```python
from build123d import *

# Parameters (mm, degrees)
F0_R     = 75.6558411923
F1_DEPTH = 48.514
F2_R     = 5.08


with BuildPart() as f1:
    # F0 (on Top) → F1 (new body)
    with BuildSketch(Plane.XY):
        Circle(F0_R)
        Polygon((0, -69.7530433536), (-46.3102683425, -29.7708865255), (41.9956482947, -29.7708865255), align=None, mode=Mode.SUBTRACT)
        with BuildLine():
            add(Edge.make_bspline(
                [(-21.8607485294, 33.7978675961), (-21.8607485294, 44.4959185344), (-39.0945518587, 45.4823768148)],
                knots=[0, 0, 0, 1.4784559967, 1.4784559967, 1.4784559967], degree=2, weights=[1, 0.73898889, 1]))
            add(Edge.make_bspline(
                [(-39.0945518587, 22.1133583775), (-21.8607485294, 23.0998166579), (-21.8607485294, 33.7978675961)],
                knots=[4.8047293104, 4.8047293104, 4.8047293104, 6.2831853072, 6.2831853072, 6.2831853072], degree=2, weights=[1, 0.73898889, 1]))
            add(Edge.make_bspline(
                [(-40.8450812101, 21.1076120934), (-39.9337015522, 21.1076120934), (-39.0945518587, 22.1133583775)],
                knots=[0, 0, 0, 0.4008066518, 0.4008066518, 0.4008066518], degree=2, weights=[1, 0.9799863696, 1]))
            add(Edge.make_bspline(
                [(-42.5956105616, 22.1133583775), (-41.7564608681, 21.1076120934), (-40.8450812101, 21.1076120934)],
                knots=[5.8823786554, 5.8823786554, 5.8823786554, 6.2831853072, 6.2831853072, 6.2831853072], degree=2, weights=[1, 0.9799863696, 1]))
            add(Edge.make_bspline(
                [(-42.5956105616, 45.4823768148), (-59.8294138908, 44.4959185344), (-59.8294138908, 33.7978675961), (-59.8294138908, 23.0998166579), (-42.5956105616, 22.1133583775)],
                knots=[1.6631366568, 1.6631366568, 1.6631366568, 3.1415926536, 3.1415926536, 4.6200486503, 4.6200486503, 4.6200486503], degree=2, weights=[1, 0.73898889, 1, 0.73898889, 1]))
            add(Edge.make_bspline(
                [(-39.0945518587, 45.4823768148), (-40.8450812101, 47.5804391797), (-42.5956105616, 45.4823768148)],
                knots=[2.7407860018, 2.7407860018, 2.7407860018, 3.5423993054, 3.5423993054, 3.5423993054], degree=2, weights=[1, 0.9207465694, 1]))
        make_face(mode=Mode.SUBTRACT)
        with BuildLine():
            add(Edge.make_bspline(
                [(21.8607485294, 33.7978675961), (21.8607485294, 23.0998166579), (39.0945518587, 22.1133583775)],
                knots=[0, 0, 0, 1.4784559967, 1.4784559967, 1.4784559967], degree=2, weights=[1, 0.73898889, 1]))
            add(Edge.make_bspline(
                [(39.0945518587, 45.4823768148), (21.8607485294, 44.4959185344), (21.8607485294, 33.7978675961)],
                knots=[4.8047293104, 4.8047293104, 4.8047293104, 6.2831853072, 6.2831853072, 6.2831853072], degree=2, weights=[1, 0.73898889, 1]))
            add(Edge.make_bspline(
                [(42.5956105616, 45.4823768148), (40.8450812101, 47.5804391797), (39.0945518587, 45.4823768148)],
                knots=[2.7407860018, 2.7407860018, 2.7407860018, 3.5423993054, 3.5423993054, 3.5423993054], degree=2, weights=[1, 0.9207465694, 1]))
            add(Edge.make_bspline(
                [(42.5956105616, 22.1133583775), (59.8294138908, 23.0998166579), (59.8294138908, 33.7978675961), (59.8294138908, 44.4959185344), (42.5956105616, 45.4823768148)],
                knots=[1.6631366568, 1.6631366568, 1.6631366568, 3.1415926536, 3.1415926536, 4.6200486503, 4.6200486503, 4.6200486503], degree=2, weights=[1, 0.73898889, 1, 0.73898889, 1]))
            add(Edge.make_bspline(
                [(40.8450812101, 21.1076120934), (41.7564608681, 21.1076120934), (42.5956105616, 22.1133583775)],
                knots=[0, 0, 0, 0.4008066518, 0.4008066518, 0.4008066518], degree=2, weights=[1, 0.9799863696, 1]))
            add(Edge.make_bspline(
                [(39.0945518587, 22.1133583775), (39.9337015522, 21.1076120934), (40.8450812101, 21.1076120934)],
                knots=[5.8823786554, 5.8823786554, 5.8823786554, 6.2831853072, 6.2831853072, 6.2831853072], degree=2, weights=[1, 0.9799863696, 1]))
        make_face(mode=Mode.SUBTRACT)
        with BuildLine():
            add(Edge.make_bspline(
                [(-39.0945518587, 22.1133583775), (-29.3455202344, 33.7978675961), (-39.0945518587, 45.4823768148)],
                knots=[0.4008066518, 0.4008066518, 0.4008066518, 2.7407860018, 2.7407860018, 2.7407860018], degree=2, weights=[1, 0.390161191, 1]))
            add(Edge.make_bspline(
                [(-39.0945518587, 45.4823768148), (-40.8450812101, 45.5825766454), (-42.5956105616, 45.4823768148)],
                knots=[1.4784559967, 1.4784559967, 1.4784559967, 1.6631366568, 1.6631366568, 1.6631366568], degree=2, weights=[1, 0.9957396602, 1]))
            add(Edge.make_bspline(
                [(-42.5956105616, 45.4823768148), (-52.3446421858, 33.7978675961), (-42.5956105616, 22.1133583775)],
                knots=[3.5423993054, 3.5423993054, 3.5423993054, 5.8823786554, 5.8823786554, 5.8823786554], degree=2, weights=[1, 0.390161191, 1]))
            add(Edge.make_bspline(
                [(-42.5956105616, 22.1133583775), (-40.8450812101, 22.0131585469), (-39.0945518587, 22.1133583775)],
                knots=[4.6200486503, 4.6200486503, 4.6200486503, 4.8047293104, 4.8047293104, 4.8047293104], degree=2, weights=[1, 0.9957396602, 1]))
        make_face()
        with BuildLine():
            add(Edge.make_bspline(
                [(-39.0945518587, 45.4823768148), (-40.8450812101, 45.5825766454), (-42.5956105616, 45.4823768148)],
                knots=[1.4784559967, 1.4784559967, 1.4784559967, 1.6631366568, 1.6631366568, 1.6631366568], degree=2, weights=[1, 0.9957396602, 1]))
            add(Edge.make_bspline(
                [(-39.0945518587, 45.4823768148), (-40.8450812101, 47.5804391797), (-42.5956105616, 45.4823768148)],
                knots=[2.7407860018, 2.7407860018, 2.7407860018, 3.5423993054, 3.5423993054, 3.5423993054], degree=2, weights=[1, 0.9207465694, 1]))
        make_face()
        with BuildLine():
            add(Edge.make_bspline(
                [(-40.8450812101, 21.1076120934), (-39.9337015522, 21.1076120934), (-39.0945518587, 22.1133583775)],
                knots=[0, 0, 0, 0.4008066518, 0.4008066518, 0.4008066518], degree=2, weights=[1, 0.9799863696, 1]))
            add(Edge.make_bspline(
                [(-42.5956105616, 22.1133583775), (-40.8450812101, 22.0131585469), (-39.0945518587, 22.1133583775)],
                knots=[4.6200486503, 4.6200486503, 4.6200486503, 4.8047293104, 4.8047293104, 4.8047293104], degree=2, weights=[1, 0.9957396602, 1]))
            add(Edge.make_bspline(
                [(-42.5956105616, 22.1133583775), (-41.7564608681, 21.1076120934), (-40.8450812101, 21.1076120934)],
                knots=[5.8823786554, 5.8823786554, 5.8823786554, 6.2831853072, 6.2831853072, 6.2831853072], degree=2, weights=[1, 0.9799863696, 1]))
        make_face()
        with BuildLine():
            add(Edge.make_bspline(
                [(39.0945518587, 45.4823768148), (29.3455202344, 33.7978675961), (39.0945518587, 22.1133583775)],
                knots=[3.5423993054, 3.5423993054, 3.5423993054, 5.8823786554, 5.8823786554, 5.8823786554], degree=2, weights=[1, 0.390161191, 1]))
            add(Edge.make_bspline(
                [(39.0945518587, 22.1133583775), (40.8450812101, 22.0131585469), (42.5956105616, 22.1133583775)],
                knots=[1.4784559967, 1.4784559967, 1.4784559967, 1.6631366568, 1.6631366568, 1.6631366568], degree=2, weights=[1, 0.9957396602, 1]))
            add(Edge.make_bspline(
                [(42.5956105616, 22.1133583775), (52.3446421858, 33.7978675961), (42.5956105616, 45.4823768148)],
                knots=[0.4008066518, 0.4008066518, 0.4008066518, 2.7407860018, 2.7407860018, 2.7407860018], degree=2, weights=[1, 0.390161191, 1]))
            add(Edge.make_bspline(
                [(42.5956105616, 45.4823768148), (40.8450812101, 45.5825766454), (39.0945518587, 45.4823768148)],
                knots=[4.6200486503, 4.6200486503, 4.6200486503, 4.8047293104, 4.8047293104, 4.8047293104], degree=2, weights=[1, 0.9957396602, 1]))
        make_face()
        with BuildLine():
            add(Edge.make_bspline(
                [(39.0945518587, 22.1133583775), (40.8450812101, 22.0131585469), (42.5956105616, 22.1133583775)],
                knots=[1.4784559967, 1.4784559967, 1.4784559967, 1.6631366568, 1.6631366568, 1.6631366568], degree=2, weights=[1, 0.9957396602, 1]))
            add(Edge.make_bspline(
                [(39.0945518587, 22.1133583775), (39.9337015522, 21.1076120934), (40.8450812101, 21.1076120934)],
                knots=[5.8823786554, 5.8823786554, 5.8823786554, 6.2831853072, 6.2831853072, 6.2831853072], degree=2, weights=[1, 0.9799863696, 1]))
            add(Edge.make_bspline(
                [(40.8450812101, 21.1076120934), (41.7564608681, 21.1076120934), (42.5956105616, 22.1133583775)],
                knots=[0, 0, 0, 0.4008066518, 0.4008066518, 0.4008066518], degree=2, weights=[1, 0.9799863696, 1]))
        make_face()
        with BuildLine():
            add(Edge.make_bspline(
                [(42.5956105616, 45.4823768148), (40.8450812101, 47.5804391797), (39.0945518587, 45.4823768148)],
                knots=[2.7407860018, 2.7407860018, 2.7407860018, 3.5423993054, 3.5423993054, 3.5423993054], degree=2, weights=[1, 0.9207465694, 1]))
            add(Edge.make_bspline(
                [(42.5956105616, 45.4823768148), (40.8450812101, 45.5825766454), (39.0945518587, 45.4823768148)],
                knots=[4.6200486503, 4.6200486503, 4.6200486503, 4.8047293104, 4.8047293104, 4.8047293104], degree=2, weights=[1, 0.9957396602, 1]))
        make_face()
    extrude(amount=F1_DEPTH)

    # F2
    f2_edges = [f1.edges().sort_by_distance(p)[0] for p in [
        (-75.655841, 0, 48.514),
    ]]
    fillet(f2_edges, radius=F2_R)


solid = f1.part
```
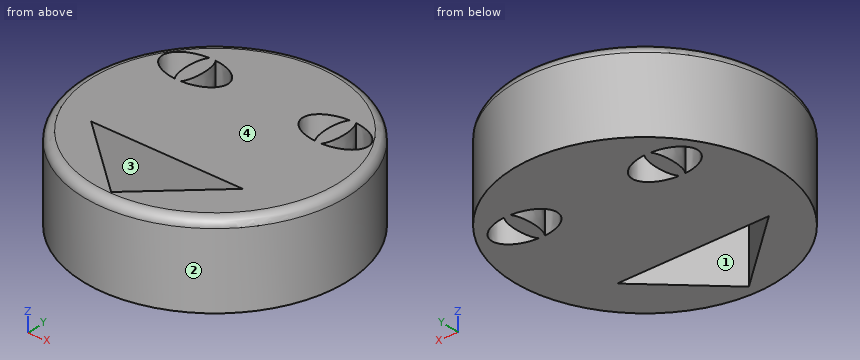
Design review of the part built by this model. Coordinates are the model's own, in mm. Face numbers are marked on the shaded views. Coordinates: 2 decimals unless noted, no trailing zeros.
1) Wall thickness on line 1 along Y through (x, z) = (-31, 33); line 2 along Y through (x, z) = (28, 32.5); line 3 along X through (y, z) = (-65, 40): over which ranges is each line inside the solid? List them lowest first.
2) Clearance check with flat-ended pins moving along their axes: pin 1 (1.5 mm diameter, centred on y = 19, z = 43.5, fed in from -X); pin 2 (1 mm diameter, centred on x = -12.5, z = 43.5, fed in from +Y); pin 3 (5 mm diameter, centred on y = 18.5, z = 13, fed in from -X). State where each tip first meets the part, or that it passes through.
3) Mouldability with a two-part tool opening along Y and no side actions: class the marked faces 1, 2, 3 and 4 as +Y half, -Y half, draft (parallel to the pull), parting line (faces both ways), or undercut.
4) Take a section at A-A, the plane z = 40.5. State how many separate pieces and enclosed holes the cut face has, and give its area (3 significant figures).
Returned:
1. line 1: y = -69.01 to -42.99, -29.77 to 23.76, 43.83 to 69.01
1. line 2: y = -70.28 to -43.1, -29.77 to 25.16, 42.44 to 70.28
1. line 3: x = -38.71 to -5.51, 4.99 to 38.71
2. pin 1: stops at x = -73.42
2. pin 2: stops at y = 74.7
2. pin 3: stops at x = -73.94
3. face 1: undercut
3. face 2: parting line
3. face 3: undercut
3. face 4: draft
4. separate pieces: 1
4. enclosed holes: 5
4. area: 15,200 mm2
